```python
from build123d import *

# Parameters (mm, degrees)
SKETCH1_W           = 203.2
SKETCH1_H           = 203.2
BOSS_EXTRUDE1_DEPTH = 6.35
FILLET1_R           = 12.7
SKETCH2_R           = 3.175
CUT_EXTRUDE1_DEPTH  = 7.35
CUT_EXTRUDE2_DEPTH  = 3.175
FILLET2_R           = 2.54
SKETCH23_R          = 3.175
CUT_EXTRUDE3_DEPTH  = 7.35


with BuildPart() as part:
    # Sketch1 → Boss-Extrude1 (new body)
    with BuildSketch(Plane(origin=(0, 0, 0), x_dir=(1, 0, 0), z_dir=(0, 1, 0))):
        with Locations((101.6, 101.6)):
            Rectangle(SKETCH1_W, SKETCH1_H)
    extrude(amount=BOSS_EXTRUDE1_DEPTH)

    # Fillet1
    fillet1_edges = [part.edges().sort_by_distance(p)[0] for p in [
        (0, 3.175, -203.2),
        (203.2, 3.175, -203.2),
        (203.2, 3.175, 0),
        (0, 3.175, 0),
    ]]
    fillet(fillet1_edges, radius=FILLET1_R)

    # Sketch2 → Cut-Extrude1 (cut, through all)
    with BuildSketch(Plane.XZ):
        with Locations((12.7, -12.7)):
            Circle(SKETCH2_R)
        with Locations((190.5, -12.7)):
            Circle(SKETCH2_R)
        with Locations((190.5, -190.5)):
            Circle(SKETCH2_R)
        with Locations((12.7, -190.5)):
            Circle(SKETCH2_R)
    extrude(amount=-CUT_EXTRUDE1_DEPTH, mode=Mode.SUBTRACT)

    # Sketch22 → Cut-Extrude2 (cut)
    with BuildSketch(Plane(origin=(0, 6.35, 0), x_dir=(1, 0, 0), z_dir=(0, 1, 0))):
        Polygon((181.654219065, 181.654219065), (172.052127253, 184.227091812), (165.022908188, 177.197872747), (167.595780935, 167.595780935), (177.197872747, 165.022908188), (184.227091812, 172.052127253), align=None)
        Polygon((18.972908188, 172.052127253), (21.545780935, 181.654219065), (31.147872747, 184.227091812), (38.177091812, 177.197872747), (35.604219065, 167.595780935), (26.002127253, 165.022908188), align=None)
        Polygon((184.227091812, 31.147872747), (181.654219065, 21.545780935), (172.052127253, 18.972908188), (165.022908188, 26.002127253), (167.595780935, 35.604219065), (177.197872747, 38.177091812), align=None)
        Polygon((21.545780935, 21.545780935), (31.147872747, 18.972908188), (38.177091812, 26.002127253), (35.604219065, 35.604219065), (26.002127253, 38.177091812), (18.972908188, 31.147872747), align=None)
    extrude(amount=-CUT_EXTRUDE2_DEPTH, mode=Mode.SUBTRACT)

    # Fillet2
    fillet2_edges = [part.edges().sort_by_distance(p)[0] for p in [
        (9.525, 0, -190.5),
        (187.325, 0, -190.5),
        (187.325, 0, -12.7),
        (9.525, 0, -12.7),
    ]]
    fillet(fillet2_edges, radius=FILLET2_R)

    # Sketch23 → Cut-Extrude3 (cut, through all)
    with BuildSketch(Plane(origin=(0, 6.35, 0), x_dir=(1, 0, 0), z_dir=(0, 1, 0))):
        with Locations((190.5, 101.6)):
            Circle(SKETCH23_R)
        with Locations((101.6, 12.7)):
            Circle(SKETCH23_R)
        with Locations((12.7, 101.6)):
            Circle(SKETCH23_R)
        with Locations((101.6, 190.5)):
            Circle(SKETCH23_R)
    extrude(amount=-CUT_EXTRUDE3_DEPTH, mode=Mode.SUBTRACT)


solid = part.part
```
CAD build for the part. Positions are in the model's coordinates, mm. A direction names the side the tool comes from. Give positions to 0.01 mm unless a question says otherwise; leave off trailing zeros. Loops run counter-clockwise (first coordinate to the right, second up) from the corner with the lowest first, then second, coordinate; pieces in that order, holes last. Notation, with made-up numbers: (-26.5, -9.75) -> (22.5, -9.75) arc R5 ccw to (22.5, -4.75) -> close; hole circle Ø5 at (16.25, 44.5). An arc over 180 degrees is marked (long way). Use a Markdown table: item, result.
1. Slice it at B-B (x = 101.6). List the corners of the cut face in (y, z) (3 decimals).
Check result:
| item | result |
|---|---|
| outline | (0, -203.2) -> (6.35, -203.2) -> (6.35, -193.675) -> (0, -193.675) -> close; (0, -187.325) -> (6.35, -187.325) -> (6.35, -15.875) -> (0, -15.875) -> close; (0, -9.525) -> (6.35, -9.525) -> (6.35, 0) -> (0, 0) -> close |
2. Which spindle directions (+Z, -Z, +X, -X, +Y, -Y) get a long thin tool onto all of the face, cutting with end or side? Do faces 4 (the cylindrical face through (10.36, 3.219, -103.746)), 5 (the flat face through (180.663, 4.785, -168.488)). Say none if no direction does.
Check result:
| item | result |
|---|---|
| face 4 | +Y, -Y |
| face 5 | +Y |
3. Wall check: L1, parallel to Z at x = 12.7, y = 4.5 (3 decimals); L2, parallel to Z at x = 101.6, y = 4.5 (3 decimals); L3, parallel to X at y = 4.85, z = -190.5 (3 decimals). Give the ranges that are in metal, low to high. Write a range as [from, to].
Check result:
| item | result |
|---|---|
| L1 | z = [-203.2, -193.675], [-187.325, -104.775], [-98.425, -15.875], [-9.525, 0] |
| L2 | z = [-203.2, -193.675], [-187.325, -15.875], [-9.525, 0] |
| L3 | x = [0, 9.525], [15.875, 98.425], [104.775, 187.325], [193.675, 203.2] |
4. Mould opens along X. For faces 1 (the cylindrical face through (199.38, 3.22, -3.62)), 2 (the cylindrical face through (187.33, 4.42, -12.56)), 3 (the flat face through (100, 6.35, -103)) say: pulls with the +X half, pulls with the -X half, needs draft (parallel to the pull), parting line crosses it, or undercut.
Check result:
| item | result |
|---|---|
| face 1 | pulls with the +X half |
| face 2 | undercut |
| face 3 | needs draft |
5. Flat gauge pins, fed straight in: pin 1 (10 mm diameter, centred on x = 190.5, z = -190.5, fed in from -Y); pin 2 (8.5 mm diameter, centred on x = 12.7, z = -12.7, fed in from -Y); pin 3 (5 mm diameter, centred on x = 12.7, z = -101.6, fed in from -Y); pin 4 (6 mm diameter, centred on x = 171, z = -171, fed in from +Y) (3 decimals). Where does each tip first touch, or does it go through?
Check result:
| item | result |
|---|---|
| pin 1 | stops at y = 0.1 |
| pin 2 | stops at y = 0.47 |
| pin 3 | passes through |
| pin 4 | stops at y = 3.175 |
6. Slice it at A-A (z = -101.6). List the corners of the cut face in (x, y) (3 decimals).
Check result:
| item | result |
|---|---|
| outline | (0, 0) -> (9.525, 0) -> (9.525, 6.35) -> (0, 6.35) -> close; (15.875, 0) -> (187.325, 0) -> (187.325, 6.35) -> (15.875, 6.35) -> close; (193.675, 0) -> (203.2, 0) -> (203.2, 6.35) -> (193.675, 6.35) -> close |
7. Slice it at C-C (y = 4.5). Give the number of separate pieces and of enclosed holes in the cut face, plus the area to 3 significant figures.
Check result:
| item | result |
|---|---|
| separate pieces | 1 |
| enclosed holes | 12 |
| area | 39,900 mm^2 |
